Verification items for this drawing (mm, ordinates from the low corner). A direction names the side the tool comes from. Round coordinates to 2 decimals unless told otherwise and drop trailing zeros. Write each loop counter-clockwise with the first axis right and the second up, starting at its lowest first coordinate (ties: lowest second). Pieces come first, ordered by that corner, then holes. Notation, with made-up numbers: (-27.75, 6) -> (30.25, 6) arc R21 ccw to (30.25, 22) -> close; hole circle Ø1 at (-2, 52.5). An arc over 180 degrees is marked (long way). One line per question, with ' | ' between items.
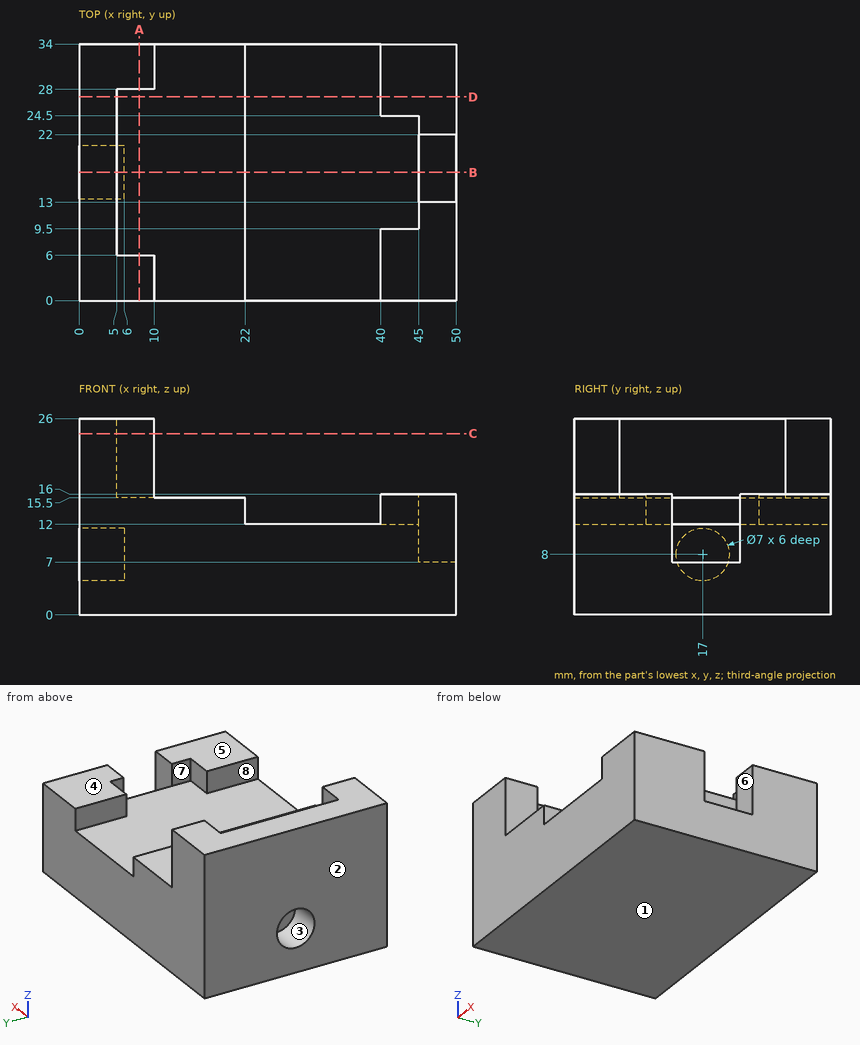
(1) Material ranges on line 1 (Z direction, x = 2.25, y = 17); line 2 (Y direction, x = 7, z = 18.75); line 3 (X direction, y = 4, z = 14.25), recorded low to high.
Resolved:
line 1: z = 0 to 4.5, 11.5 to 26 | line 2: y = 0 to 6, 28 to 34 | line 3: x = 0 to 22, 40 to 50
(2) Access from +Z, -Z, +X, -X, +Y, -Y to the whole of each face (thin tool, end or side, straight path). Record for the marked faces 5, 6, 7 and 8.
Resolved:
face 5: +Z, +X, +Y, -Y | face 6: +Z, +X | face 7: +Z | face 8: +Z, +Y, -Y
(3) Sectioned sample at D-D on y = 27. Record the cut outline in (x, z).
Resolved:
outline: (0, 0) -> (50, 0) -> (50, 16) -> (40, 16) -> (40, 12) -> (22, 12) -> (22, 15.5) -> (5, 15.5) -> (5, 26) -> (0, 26) -> close
(4) Draft check along Z on the marked faces 1, 2, 3 and 4. Enter one of: +Z half, -Z half, draft (parallel to the pull), parting line (faces both ways), or undercut.
Resolved:
face 1: -Z half | face 2: draft | face 3: undercut | face 4: +Z half
(5) Sectioned sample at A-A on x = 8. Record the cut outline in (y, z).
Resolved:
outline: (0, 0) -> (34, 0) -> (34, 26) -> (28, 26) -> (28, 15.5) -> (6, 15.5) -> (6, 26) -> (0, 26) -> close
(6) Sectioned sample at B-B on y = 17. Record the cut outline in (x, z), then the cut area to 4 significant figures.
Resolved:
outline: (0, 0) -> (50, 0) -> (50, 7) -> (45, 7) -> (45, 12) -> (22, 12) -> (22, 15.5) -> (5, 15.5) -> (5, 26) -> (0, 26) -> (0, 11.5) -> (6, 11.5) -> (6, 4.5) -> (0, 4.5) -> close | area: 662.5 mm2
(7) Go/stop test with flat-tipped pins: pin 1 (10 mm diameter, centred on x = 34.5, y = 13.5, fed in from +Z); pin 2 (3 mm diameter, centred on y = 31.5, z = 22.5, fed in from +X); pin 3 (5.5 mm diameter, centred on y = 17, z = 10, fed in from +X). Record where each tip stops, or that it passes through.
Resolved:
pin 1: stops at z = 12 | pin 2: stops at x = 10 | pin 3: stops at x = 45
(8) Sectioned sample at C-C on z = 24. Record the cut outline in (x, y), then the cut area to 3 significant figures.
Resolved:
outline: (0, 0) -> (10, 0) -> (10, 6) -> (5, 6) -> (5, 28) -> (10, 28) -> (10, 34) -> (0, 34) -> close | area: 230 mm2
